Design review of the part built by this model. Coordinates are the model's own, in mm. A direction names the side the tool comes from. Coordinates: 2 decimals unless noted, no trailing zeros. Write each loop counter-clockwise with the first axis right and the second up, starting at its lowest first coordinate (ties: lowest second). Pieces come first, ordered by that corner, then holes. Notation, with made-up numbers: (8.5, 13) - (56.5, 13) arc R19 cw to (56.5, 20) - close; hole circle Ø5 at (32, 20). An arc over 180 degrees is marked (long way). Answer as a JSON object with one key per item and string values.
```python
from build123d import *

# Parameters (mm, degrees)
F0_R      = 14.5
F1_DEPTH  = 50
F2_DEPTH  = 2
F3_R      = 50
F3_R_2    = 3
F4_DEPTH  = 6
F6_DEPTH  = 35
F7_SIZE   = 30
F8_COUNT  = 4
F10_R     = 1.5
F11_DEPTH = 30


with BuildPart() as f1:
    # F0 (on Top) → F1 (new body)
    with BuildSketch(Plane.XY):
        with BuildLine():
            ThreePointArc((19.475849062, -0.970207871), (19.4939613305, -0.4852542068), (19.5, 0))
            ThreePointArc((19.5, 0), (16.9843331812, 9.5803145245), (10.0864178063, 16.6887439862))
            ThreePointArc((10.0864178063, 16.6887439862), (10.0432424607, 16.7147623637), (10, 16.7406690428))
            ThreePointArc((10, 16.7406690428), (0, 19.5), (-10, 16.7406690428))
            ThreePointArc((-10, 16.7406690428), (-10.0432424607, -16.7147623637), (19.475849062, -0.970207871))
        make_face()
        Circle(F0_R, mode=Mode.SUBTRACT)
    extrude(amount=F1_DEPTH)

    # F0 (on Top) → F2 (join)
    with BuildSketch(Plane.XY):
        Circle(F0_R)
    extrude(amount=F2_DEPTH)

    # F3 (on Top) → F4 (join)
    with BuildSketch(Plane.XY):
        Circle(F3_R)
        with Locations((-23.5907118767, -30.2173215896)):
            Circle(F3_R_2, mode=Mode.SUBTRACT)
        with Locations((30.2173215896, -23.5907118767)):
            Circle(F3_R_2, mode=Mode.SUBTRACT)
        with Locations((-30.2173215896, 23.5907118767)):
            Circle(F3_R_2, mode=Mode.SUBTRACT)
        with Locations((23.5907118767, 30.2173215896)):
            Circle(F3_R_2, mode=Mode.SUBTRACT)
    extrude(amount=F4_DEPTH)

    # F5 (on face) → F6 (join)
    with BuildSketch(Plane.XY.offset(6)):
        with BuildLine():
            Line((4, 19.085334684), (4, 49.8397431775))
            ThreePointArc((4, 49.8397431775), (0, 50), (-4, 49.8397431775))
            Line((-4, 49.8397431775), (-4, 19.085334684))
            ThreePointArc((-4, 19.085334684), (0, 19.5), (4, 19.085334684))
        make_face()
    extrude(amount=F6_DEPTH)

    # F7
    f7_edges = [f1.edges().sort_by_distance(p)[0] for p in [
        (0, 50, 41),
    ]]
    chamfer(f7_edges, length=F7_SIZE)

    # F8: F1 ×4 about axis
    f8_axis = Axis((0, 0, 0), (0, 0, -1))


with BuildPart() as f1_1:
    add(f1.part)
    for i in range(1, F8_COUNT):
        add(f1.part.rotate(f8_axis, i * 360 / F8_COUNT))

    # F10 (on face) → F11 (cut)
    with BuildSketch(Plane(origin=(0, 0, 0), x_dir=(0.7071067812, -0.7071067812, 0), z_dir=(-0.7071067812, -0.7071067812, 0))):
        with Locations((0, 40.1646271348)):
            Circle(F10_R)
    extrude(amount=-F11_DEPTH, mode=Mode.SUBTRACT)


solid = f1_1.part
```
(1) Take a section at A-A, the plane z = 47. Write out the cut boundary in (x, y), and give its area (3 significant figures).
Solved:
{"outline": "(-16.74, 10) arc R19.5 ccw to (-10.09, -16.69) arc R19.5 ccw to (-10, -16.74) arc R19.5 ccw to (16.69, -10.09) arc R19.5 ccw to (16.74, -10) arc R19.5 ccw to (10.09, 16.69) arc R19.5 ccw to (10, 16.74) arc R19.5 ccw to (-16.69, 10.09) arc R19.5 ccw to start; hole circle Ø29 at (0, 0)", "area": "534 mm^2"}
(2) The part is to be moulded in two halves that separate along X. For faces 1 (the face through (0, 31, 30)), 2 (the face through (-33.214, 23.723, 2.958)), 3 (the face through (-4, -31, 19)), 4 (the face through (6.691, -12.864, 27.692)), say which applies: pulls with the +X half, pulls with the -X half, needs draft (parallel to the pull), parting line crosses it, or undercut.
Solved:
{"face 1": "parting line crosses it", "face 2": "undercut", "face 3": "pulls with the -X half", "face 4": "undercut"}
(3) Tool access review of faces 5 (the face through (27, -27, 6)), 6 (the face through (-31, 4, 19)), 7 (the face through (0, 0, 6)): name each direction out of +Z, -Z, +X, -X, +Y, -Y from which nothing blocks a thin tool from reaching the whole face with its end or side.
Solved:
{"face 5": "+Z, +X, -Y", "face 6": "+Z, -X, +Y", "face 7": "+Z"}
(4) To check wall thickness, follow line 1 (Z direction, x = -12, y = -25.5); line 2 (Y direction, x = 43.5, z = 13). State the ranges of each line that lie inside material, in increasing order. Write a range as from..to.
Solved:
{"line 1": "z = 0..6", "line 2": "y = -4..4"}
(5) Take a section at C-C, the plane z = 4. Write out the cut boundary in (x, y).
Solved:
{"outline": "circle Ø100 at (0, 0); hole circle Ø6 at (-30.22, 23.59); hole circle Ø6 at (-23.59, -30.22); hole circle Ø6 at (23.59, 30.22); hole circle Ø6 at (30.22, -23.59)"}
(6) For pin 1 (5 mm diameter, centred on x = 39.5, y = -30, fed in from +Z); pin 2 (3 mm diameter, centred on x = 14, y = -7.5, fed in from -Z); pin 3 (8 mm diameter, centred on x = -17.5, z = 32.5, fed in from -Y); pin 4 (9 mm diameter, centred on x = 31, z = 22.5, fed in from -Y), all flat-tipped, find the tip position at first contact; note any pin that passes through.
Solved:
{"pin 1": "stops at z = 6", "pin 2": "stops at z = 0", "pin 3": "stops at y = -14.07", "pin 4": "stops at y = -4"}
